Autodesk Inventor part; units mm, degrees
ref_plane "YZ Plane" through (0, 0, 0) normal (1, 0, 0) x (0, 1, 0)
ref_plane "XZ Plane" through (0, 0, 0) normal (0, 1, 0) x (-1, 0, 0)
ref_plane "XY Plane" through (0, 0, 0) normal (0, 0, 1) x (1, 0, 0)
sketch "Sketch1" plane through (0, 0, 0) normal (0, 0, 1) x (1, 0, 0)
  line L0 (-10, 60) -> (10, 60)
  line L1 (20, 50) -> (20, -50)
  line L2 (10, -60) -> (-10, -60)
  line L3 (-20, -50) -> (-20, 50)
  arc A0 (-10, 60) -> (-20, 50) centre (-10, 50) ccw
  arc A1 (20, 50) -> (10, 60) centre (10, 50) ccw
  arc A2 (10, -60) -> (20, -50) centre (10, -50) ccw
  arc A3 (-20, -50) -> (-10, -60) centre (-10, -50) ccw
  point P0 (0, 0)
  point P1 (20, 0)
  point P2 (0, 60)
  dimension "d0" = 10
  dimension "d1" = 40
  dimension "d2" = 120
extrude "Extrusion1" add sketch "Sketch1" along normal blind 5
sketch "Sketch2" plane through (0, 0, 5) normal (0, 0, 1) x (1, 0, 0)
  circle A0 centre (0, 50) radius 5
  line L0 (-20, 50) -> (-20, -50) construction
  line L1 (-20, 0) -> (20, 0) construction
  line L2 (20, -50) -> (20, 50) construction
  line L3 (10, 60) -> (-10, 60)
  circle A1 centre (0, -50) radius 5
  circle A2 centre (0, 0) radius 5
  point P0 (0, 0)
  dimension "d5" = 10
  dimension "d7" = 10
  dimension "d8" = 10
extrude "Extrusion2" cut sketch "Sketch2" against normal up to surface (5 mm away)
properties part number "mitad"
Work out the finished part from the listing and answer in its coordinate system (mm). Round coordinates to 2 decimals unless told otherwise and drop trailing zeros. Write each loop counter-clockwise with the first axis right and the second up, starting at its lowest first coordinate (ties: lowest second). Pieces come first, ordered by that corner, then holes. Notation, with made-up numbers: (16.5, -11.5) -> (49.5, -11.5) arc R12 ccw to (49.5, 9.5) -> close; hole circle Ø6 at (19, 58.25). An arc over 180 degrees is marked (long way). Write each question's results on one line, items separated by ' | '.
Q1. Straight lines are drawn through the part: line 1 along Y through (x, z) = (0, 2.25); line 2 along Y through (x, z) = (-4.5, 4.1); line 3 along Y through (x, z) = (-10.5, 4). For each, find the intervals that lie inside material, in ascending order. Write a range as [from, to].
Data:
line 1: [-60, -55], [-45, -5], [5, 45], [55, 60] | line 2: [-60, -52.18], [-47.82, -2.18], [2.18, 47.82], [52.18, 60] | line 3: [-59.99, 59.99]
Q2. Section C-C, the plane x = 0 is taken. Write down the section's boundary in (y, z).
Data:
outline: (-60, 0) -> (-55, 0) -> (-55, 5) -> (-60, 5) -> close; (-45, 0) -> (-5, 0) -> (-5, 5) -> (-45, 5) -> close; (5, 0) -> (45, 0) -> (45, 5) -> (5, 5) -> close; (55, 0) -> (60, 0) -> (60, 5) -> (55, 5) -> close
Q3. Section A-A, the plane y = 0 is taken. Write down the section's boundary in (x, z).
Data:
outline: (-20, 0) -> (-5, 0) -> (-5, 5) -> (-20, 5) -> close; (5, 0) -> (20, 0) -> (20, 5) -> (5, 5) -> close
Q4. Flat-ended cylindrical pins translate along their axes: P1, Ø2, axis at x = 12.5, z = 3, coming from the -Y side; P2, Ø2, axis at x = 2, y = 1.5, coming from the -Z side. Find the tip coordinate at first contact, or state that the pin passes through.
Data:
P1: y = -59.89 | P2: through
Q5. Section B-B, the plane z = 1.4 is taken. Write down the section's boundary in (x, y), then the cut area to 3 significant figures.
Data:
outline: (-20, -50) arc R10 ccw to (-10, -60) -> (10, -60) arc R10 ccw to (20, -50) -> (20, 50) arc R10 ccw to (10, 60) -> (-10, 60) arc R10 ccw to (-20, 50) -> close; hole circle Ø10 at (0, -50); hole circle Ø10 at (0, 0); hole circle Ø10 at (0, 50) | area: 4,480 mm^2
Q6. Determine the mould class of faces 1 (the flat face through (0, 60, 2)), 2 (the cylindrical face through (-0.651, -45.043, 2.535)), 3 (the cylindrical face through (17.15, -56.99, 2.46)) for opening direction Y: released by +Y, released by -Y, zero draft, split by the parting line, or undercut.
Data:
face 1: released by +Y | face 2: undercut | face 3: released by -Y
Q7. Section D-D, the plane x = 16.5 is taken. Write down the section's boundary in (y, z), then the cut area to 3 significant figures.
Data:
outline: (-57.6, 0) -> (57.6, 0) -> (57.6, 5) -> (-57.6, 5) -> close | area: 576 mm^2
